Part model, mm, in its own coordinate system. A direction names the side the tool comes from. Round coordinates to 2 decimals unless told otherwise and drop trailing zeros. Order: outer loops, then holes, each group sorted by start corner. A loop starts at its lowest first (then second) coordinate and runs counter-clockwise, first axis right, second up. Notation, with made-up numbers: (-36.75, -27) - (-25.75, -27) arc R26 ccw to (-25.75, -9) - close; hole circle Ø7 at (77.25, 3.25). An arc over 180 degrees is marked (long way). Return JSON: item names as keys, results as strings. Group by question number.
Item 1: Saw through at B-B on y = 3.81. List the corners of the cut face in (x, z) (3 decimals), and give its area (3 significant figures).
Item 2: Saw through at A-A on y = 38.1. List the corners of the cut face in (x, z) (3 decimals), and give its area (3 significant figures).
Item 3: Saw through at C-C on x = 23. List the corners of the cut face in (y, z), and give its area (3 significant figures).
Item 4: Saw through at D-D on z = 5. State how many separate pieces and enclosed holes the cut face has, and give its area (3 significant figures).
Item 5: Tool access for faces 1 (the face through (35.78, 0.9, 3.22)), 2 (the face through (27, 32, 6.35)): list every direction of +Z, -Z, +X, -X, +Y, -Y with a clear straight run to the whole face (end or side of a thin tool).
Item 6: Drop flat-ended pins along their axis: pin 1 (2.5 mm diameter, centred on x = 2.43, y = 3.81, fed in from +Z) (1 decimal); pin 2 (12 mm diameter, centred on x = 26, y = 39.5, fed in from -Z). Give the stop position or say it passes through.
Item 7: Probe probe 1 along X at (y, z) = (49.5, 1.5); probe 2 along X at (y, z) = (6.5, 1.25) (3 decimals); probe 3 along Y at (x, z) = (39.5, 4.5). List the from-to ranges inside material, lowest first.
Item 8: Two-plate mould, pull along Y, no slides. Class faces 3 (the face through (8.623, 0.855, 3.219)), 4 (the face through (40.524, 3.876, 3.131)), 5 (the face through (5.332, 16.631, 3.131)), 6 (the face through (0, 27, 3)): released by +Y, released by -Y, zero draft, split by the parting line, or undercut.
```python
from build123d import *

# Parameters (mm, degrees)
SKETCH1_R           = 1.5875
SKETCH1_R_2         = 1.65
SKETCH1_R_3         = 1.5
BOSS_EXTRUDE1_DEPTH = 6.35
FILLET1_R           = 3


with BuildPart() as part:
    # Sketch1 → Boss-Extrude1 (new body)
    with BuildSketch(Plane.XY):
        with BuildLine():
            Line((0, 0), (9.525, 0))
            Line((9.525, 0), (9.525, 15.24))
            ThreePointArc((9.525, 15.24), (22.225, 27.94), (34.925, 15.24))
            Line((34.925, 15.24), (34.925, 0))
            Line((34.925, 0), (44.45, 0))
            Line((44.45, 0), (44.45, 52.563))
            Line((44.45, 52.563), (0, 52.563))
            Line((0, 52.563), (0, 0))
        make_face()
        with Locations((5.715, 49.388)):
            Circle(SKETCH1_R, mode=Mode.SUBTRACT)
        with Locations((38.735, 49.388)):
            Circle(SKETCH1_R, mode=Mode.SUBTRACT)
        with Locations((4.445, 15.24)):
            Circle(SKETCH1_R_2, mode=Mode.SUBTRACT)
        with Locations((22.225, 33.02)):
            Circle(SKETCH1_R_2, mode=Mode.SUBTRACT)
        with Locations((40.005, 15.24)):
            Circle(SKETCH1_R_2, mode=Mode.SUBTRACT)
        with Locations((22.225, 38.1)):
            Circle(SKETCH1_R_3, mode=Mode.SUBTRACT)
        with Locations((42.022340731, 3.81)):
            Circle(SKETCH1_R_3, mode=Mode.SUBTRACT)
        with Locations((2.427659269, 3.81)):
            Circle(SKETCH1_R_3, mode=Mode.SUBTRACT)
    extrude(amount=BOSS_EXTRUDE1_DEPTH)

    # Fillet1
    fillet1_edges = [part.edges().sort_by_distance(p)[0] for p in [
        (9.525, 0, 3.175),
        (0, 0, 3.175),
        (0, 52.563, 3.175),
        (44.45, 52.563, 3.175),
        (44.45, 0, 3.175),
        (34.925, 0, 3.175),
    ]]
    fillet(fillet1_edges, radius=FILLET1_R)


solid = part.part
```
Filled in:
{
 "1": {"outline": "(0, 0) - (0.928, 0) - (0.928, 6.35) - (0, 6.35) - close; (3.928, 0) - (9.525, 0) - (9.525, 6.35) - (3.928, 6.35) - close; (34.925, 0) - (40.522, 0) - (40.522, 6.35) - (34.925, 6.35) - close; (43.522, 0) - (44.45, 0) - (44.45, 6.35) - (43.522, 6.35) - close", "area": "82.9 mm^2"},
 "2": {"outline": "(0, 0) - (20.725, 0) - (20.725, 6.35) - (0, 6.35) - close; (23.725, 0) - (44.45, 0) - (44.45, 6.35) - (23.725, 6.35) - close", "area": "263 mm^2"},
 "3": {"outline": "(27.92, 0) - (31.56, 0) - (31.56, 6.35) - (27.92, 6.35) - close; (34.48, 0) - (36.82, 0) - (36.82, 6.35) - (34.48, 6.35) - close; (39.38, 0) - (52.56, 0) - (52.56, 6.35) - (39.38, 6.35) - close", "area": "122 mm^2"},
 "4": {"separate pieces": "1", "enclosed holes": "8", "area": "1,620 mm^2"},
 "5": {"face 1": "+Z, -Z, -Y", "face 2": "+Z, +X, -X, +Y, -Y"},
 "6": {"pin 1": "passes through", "pin 2": "stops at z = 0"},
 "7": {"probe 1": "x = 0 to 4.13, 7.3 to 37.15, 40.32 to 44.45", "probe 2": "x = 0 to 9.525, 34.925 to 44.45", "probe 3": "y = 0 to 13.67, 16.81 to 48, 50.78 to 52.56"},
 "8": {"face 3": "released by -Y", "face 4": "undercut", "face 5": "undercut", "face 6": "zero draft"}
}
